```python
from build123d import *

# Parameters (mm, degrees)
CROQUIS2_W              = 6.5
CROQUIS2_H              = 6.5
SALIENTE_EXTRUIR1_DEPTH = 85
REDONDEO1_R             = 3
CHAFL_N1_SIZE           = 1


with BuildPart() as part:
    # Croquis2 → Saliente-Extruir1 (new body)
    with BuildSketch(Plane(origin=(0, 0, 0), x_dir=(0, 0, -1), z_dir=(1, 0, 0))):
        with Locations((-3.25, 3.25)):
            Rectangle(CROQUIS2_W, CROQUIS2_H)
    extrude(amount=SALIENTE_EXTRUIR1_DEPTH)

    # Redondeo1
    redondeo1_edges = [part.edges().sort_by_distance(p)[0] for p in [
        (42.5, 0, 6.5),
        (42.5, 6.5, 6.5),
    ]]
    fillet(redondeo1_edges, radius=REDONDEO1_R)

    # Chaflán1
    chafl_n1_edges = [part.edges().sort_by_distance(p)[0] for p in [
        (0, 0, 1.75),
        (85, 0, 1.75),
        (0, 3.25, 6.5),
        (0, 5.621320344, 5.621320344),
        (0, 0.878679656, 5.621320344),
        (85, 3.25, 6.5),
        (85, 5.621320344, 5.621320344),
        (85, 0.878679656, 5.621320344),
        (0, 6.5, 1.75),
        (85, 6.5, 1.75),
        (42.5, 0, 0),
        (42.5, 6.5, 0),
    ]]
    chamfer(chafl_n1_edges, length=CHAFL_N1_SIZE)


solid = part.part
```
Verification items for the finished model (mm, model axes). Give positions to 0.01 mm unless a question says otherwise; leave off trailing zeros. Loops run counter-clockwise (first coordinate to the right, second up) from the corner with the lowest first, then second, coordinate; pieces in that order, holes last. Notation, with made-up numbers: M 22,-28 L 37,-28 A5 ccw 37,-21 Z; hole C 39,72 d6. An arc over 180 degrees is marked long. One line per question, with ' | ' between items.
Item 1: Section check A-A, the plane x = 58. Record the cut outline in (y, z), plus the area to 3 significant figures.
Completed:
outline: M 0,1 L 1,0 L 5.5,0 L 6.5,1 L 6.5,3.5 A3 ccw 3.5,6.5 L 3,6.5 A3 ccw 0,3.5 Z | area: 37.4 mm^2
Item 2: Thickness scan on line 1 (Z direction, x = 73, y = 3.75); line 2 (X direction, y = 3.75, z = 5.5); line 3 (Z direction, x = 14.5, y = 4.5). Record the ranges inside material, lowest first. Write a range as [from, to].
Completed:
line 1: z = [0, 6.49] | line 2: x = [0.02, 84.98] | line 3: z = [0, 6.33]
Item 3: Draft check along X on faces 1 (the face through (0.4, 1.32, 5.21)), 2 (the face through (85, 3, 3)), 3 (the face through (42, 3, 0)). Enter one of: +X half, -X half, draft (parallel to the pull), parting line (faces both ways), or undercut.
Completed:
face 1: -X half | face 2: +X half | face 3: draft
Item 4: Depth check by flat-ended pin: P1, Ø1, axis at x = 26.5, y = 4.5, coming from the -Z side. Enter the tip coordinate at first touch or a pass-through.
Completed:
P1: stops at z = 0
